Geometry check sheet. Reference: the model listing, model coordinates, mm. A direction names the side the tool comes from. Round coordinates to 2 decimals unless told otherwise and drop trailing zeros. Write each loop counter-clockwise with the first axis right and the second up, starting at its lowest first coordinate (ties: lowest second). Pieces come first, ordered by that corner, then holes. Notation, with made-up numbers: (-26, 24) - (-1, 24) arc R12 ccw to (-1, 37) - close; hole circle Ø9 at (80.5, 43.25). An arc over 180 degrees is marked (long way). Return JSON: item names as keys, results as strings.
```python
from build123d import *

# Parameters (mm, degrees)
F0_W     = 93
F0_H     = 65
F1_DEPTH = 3
F2_R     = 5
F3_R     = 2


with BuildPart() as f1:
    # F0 (on Top) → F1 (new body)
    with BuildSketch(Plane.XY):
        Rectangle(F0_W, F0_H)
        with BuildLine():
            Line((-39.5, -10.5), (-39.5, 7.5))
            ThreePointArc((-39.5, 7.5), (-38.5, 8.5), (-37.5, 7.5))
            Line((-37.5, 7.5), (-37.5, -10.5))
            ThreePointArc((-37.5, -10.5), (-38.5, -11.5), (-39.5, -10.5))
        make_face(mode=Mode.SUBTRACT)
        with BuildLine():
            Line((2, -6), (2, -26))
            ThreePointArc((2, -26), (1, -27), (0, -26))
            Line((0, -26), (0, -6))
            ThreePointArc((0, -6), (1, -5), (2, -6))
        make_face(mode=Mode.SUBTRACT)
    extrude(amount=F1_DEPTH)

    # F2
    f2_edges = [f1.edges().sort_by_distance(p)[0] for p in [
        (-46.5, 32.5, 1.5),
        (-46.5, -32.5, 1.5),
    ]]
    fillet(f2_edges, radius=F2_R)

    # F3
    f3_edges = [f1.edges().sort_by_distance(p)[0] for p in [
        (46.5, -32.5, 1.5),
        (46.5, 32.5, 1.5),
    ]]
    fillet(f3_edges, radius=F3_R)


solid = f1.part
```
(1) Release check for a two-part mould opening along X. For faces 3 (the face through (-37.5, -1, 1)), 4 (the face through (-1, 0, 0)), 5 (the face through (-46.5, 0, 1)), 6 (the face through (46.5, 0, 1)) record: pulls with the +X half, pulls with the -X half, needs draft (parallel to the pull), parting line crosses it, or undercut.
Response values:
{"face 3": "undercut", "face 4": "needs draft", "face 5": "pulls with the -X half", "face 6": "pulls with the +X half"}
(2) Material ranges on line 1 along X through (y, z) = (-9, 1.35); line 2 along X through (y, z) = (5, 0.4); line 3 along X through (y, z) = (-16, 1.6), recorded low to high. Write a range as [from, to].
Response values:
{"line 1": "x = [-46.5, -39.5], [-37.5, 0], [2, 46.5]", "line 2": "x = [-46.5, -39.5], [-37.5, 46.5]", "line 3": "x = [-46.5, 0], [2, 46.5]"}
(3) Section check B-B, the plane z = 2.4. Enter the section's corners in (x, y).
Response values:
{"outline": "(-46.5, -27.5) arc R5 ccw to (-41.5, -32.5) - (44.5, -32.5) arc R2 ccw to (46.5, -30.5) - (46.5, 30.5) arc R2 ccw to (44.5, 32.5) - (-41.5, 32.5) arc R5 ccw to (-46.5, 27.5) - close; hole (-39.5, -10.5) arc R1 ccw to (-37.5, -10.5) - (-37.5, 7.5) arc R1 ccw to (-39.5, 7.5) - close; hole (0, -26) arc R1 ccw to (2, -26) - (2, -6) arc R1 ccw to (0, -6) - close"}
(4) Section check A-A, the plane x = -38.5. Enter the section's corners in (y, z).
Response values:
{"outline": "(-32.5, 0) - (-11.5, 0) - (-11.5, 3) - (-32.5, 3) - close; (8.5, 0) - (32.5, 0) - (32.5, 3) - (8.5, 3) - close"}
(5) Access from +Z, -Z, +X, -X, +Y, -Y to the whole of each face (thin tool, end or side, straight path). Record for faces 1 (the face through (45.9, -31.93, 1.52)), 2 (the face through (0, -16, 1)).
Response values:
{"face 1": "+Z, -Z, +X, -Y", "face 2": "+Z, -Z"}
(6) Section check C-C, the plane y = -3. Enter the section's corners in (x, z).
Response values:
{"outline": "(-46.5, 0) - (-39.5, 0) - (-39.5, 3) - (-46.5, 3) - close; (-37.5, 0) - (46.5, 0) - (46.5, 3) - (-37.5, 3) - close"}
